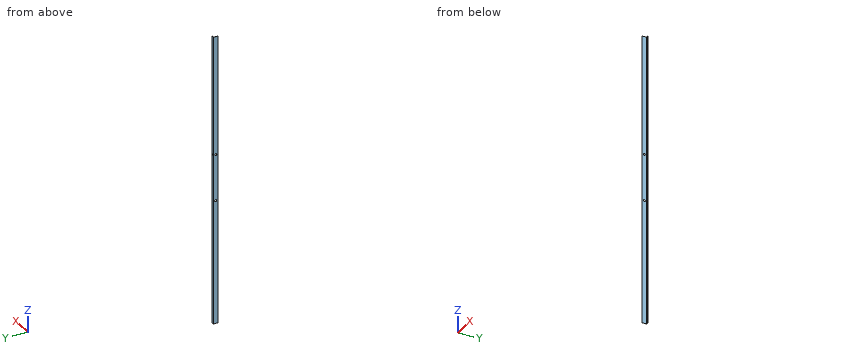
from build123d import *

# Parameters (mm, degrees)
F0_W     = 0.5
F0_H     = 19.5
F0_H_2   = 0.5
F0_W_2   = 9.5
F1_DEPTH = 1300
F2_R     = 4.5
F3_DEPTH = 25
F4_R     = 2.5
F5_DEPTH = 25
F6_R     = 4.5
F7_DEPTH = 25


with BuildPart() as f1:
    # F0 (on Top) → F1 (new body)
    with BuildSketch(Plane.XY):
        with Locations((-56.969816, -30.547241)):
            Rectangle(F0_W, F0_H)
        with Locations((-56.969816, -20.547241)):
            Rectangle(F0_W, F0_H_2)
        with Locations((-51.969816, -20.547241)):
            Rectangle(F0_W_2, F0_H_2)
    extrude(amount=F1_DEPTH)

    # F2 (on face) → F3 (cut)
    with BuildSketch(Plane(origin=(-57.219816, 0, 0), x_dir=(0, -1, 0), z_dir=(-1, 0, 0))):
        with Locations((31.05364, 765.408933)):
            Circle(F2_R)
    extrude(amount=-F3_DEPTH, mode=Mode.SUBTRACT)

    # F4 (on face) → F5 (cut)
    with BuildSketch(Plane(origin=(0, -20.297241, 0), x_dir=(-1, 0, 0), z_dir=(0, 1, 0))):
        with Locations((52.001603, 765.470803)):
            Circle(F4_R)
    extrude(amount=-F5_DEPTH, mode=Mode.SUBTRACT)

    # F6 (on face) → F7 (cut)
    with BuildSketch(Plane(origin=(-57.219816, 0, 0), x_dir=(0, -1, 0), z_dir=(-1, 0, 0))):
        with Locations((30.562836, 556.409509)):
            Circle(F6_R)
    extrude(amount=-F7_DEPTH, mode=Mode.SUBTRACT)


solid = f1.part
Part model, mm, in its own coordinate system. Give positions to 0.01 mm unless a question says otherwise; leave off trailing zeros. Loops run counter-clockwise (first coordinate to the right, second up) from the corner with the lowest first, then second, coordinate; pieces in that order, holes last. Notation, with made-up numbers: M 24.25,16 L 74.25,16 A18 cw 74.25,24 Z; hole C -23.5,-28.5 d9. An arc over 180 degrees is marked long. Put each result on its own line as item: value. Start each with the question number.
1) Saw through at C-C (z = 478.5). List the corners of the cut face in (x, y).
2) Probe probe 1 along Y at (x, z) = (-47.75, 93); probe 2 along X at (y, z) = (-37.5, 762). List the from-to ranges inside material, lowest first.
3) Saw through at A-A (x = -51.25). List the corners of the cut face in (y, z).
4) Saw through at B-B (y = -30.5). List the corners of the cut face in (x, z).
5) Flat gauge pins, fed straight in: pin 1 (1 mm diameter, centred on x = -51, z = 821.5, fed in from -Y); pin 2 (8 mm diameter, centred on y = -29.5, z = 688.5, fed in from +X); pin 3 (10 mm diameter, centred on y = -22.5, z = 935.5, fed in from +X). Where does each tip first touch, or does it go through?
Numbers:
1. outline: M -57.22,-40.3 L -56.72,-40.3 L -56.72,-20.8 L -47.22,-20.8 L -47.22,-20.3 L -57.22,-20.3 Z
2. probe 1: -20.8 to -20.3
2. probe 2: -57.22 to -56.72
3. outline: M -20.8,0 L -20.3,0 L -20.3,763.09 L -20.8,763.09 Z; M -20.8,767.86 L -20.3,767.86 L -20.3,1300 L -20.8,1300 Z
4. outline: M -57.22,0 L -56.72,0 L -56.72,551.91 L -57.22,551.91 Z; M -57.22,560.91 L -56.72,560.91 L -56.72,760.94 L -57.22,760.94 Z; M -57.22,769.87 L -56.72,769.87 L -56.72,1300 L -57.22,1300 Z
5. pin 1: y = -20.8
5. pin 2: x = -56.72
5. pin 3: x = -47.22
